The model under review builds one solid part; all positions refer to its coordinate system, in mm. Face numbers are marked on the shaded views. A direction names the side the tool comes from. Round coordinates to 2 decimals unless told otherwise and drop trailing zeros. Order: outer loops, then holes, each group sorted by start corner. A loop starts at its lowest first (then second) coordinate and runs counter-clockwise, first axis right, second up.
```python
from build123d import *

# Parameters (mm, degrees)
F1_DEPTH = 12
F3_DEPTH = 10
F4_W     = 12
F4_H     = 7.5
F5_DEPTH = 10


with BuildPart() as f1:
    # F0 (on Top) → F1 (new body)
    with BuildSketch(Plane.XY):
        with BuildLine():
            Line((-12.672, -19.5), (11.5, -19.5))
            ThreePointArc((11.5, -19.5), (17.156854, -17.156854), (19.5, -11.5))
            Line((19.5, -11.5), (19.5, 11.5))
            ThreePointArc((19.5, 11.5), (17.156854, 17.156854), (11.5, 19.5))
            Line((11.5, 19.5), (-12.672, 19.5))
            ThreePointArc((-12.672, 19.5), (-17.500125, 17.500125), (-19.5, 12.672))
            Line((-19.5, 12.672), (-19.5, -12.672))
            ThreePointArc((-19.5, -12.672), (-17.500125, -17.500125), (-12.672, -19.5))
        make_face()
    extrude(amount=F1_DEPTH)

    # F2 (on face) → F3 (cut)
    with BuildSketch(Plane.XY.offset(12)):
        with BuildLine():
            Line((-10.672, -17.5), (9.5, -17.5))
            ThreePointArc((9.5, -17.5), (15.156854, -15.156854), (17.5, -9.5))
            Line((17.5, -9.5), (17.5, 9.5))
            ThreePointArc((17.5, 9.5), (15.156854, 15.156854), (9.5, 17.5))
            Line((9.5, 17.5), (-10.672, 17.5))
            ThreePointArc((-10.672, 17.5), (-15.500125, 15.500125), (-17.5, 10.672))
            Line((-17.5, 10.672), (-17.5, -10.672))
            ThreePointArc((-17.5, -10.672), (-15.500125, -15.500125), (-10.672, -17.5))
        make_face()
    extrude(amount=-F3_DEPTH, mode=Mode.SUBTRACT)

    # F4 (on face) → F5 (cut)
    with BuildSketch(Plane.YZ.offset(19.5)):
        with Locations((-5.2, 5.004)):
            Rectangle(F4_W, F4_H)
    extrude(amount=-F5_DEPTH, mode=Mode.SUBTRACT)


solid = f1.part
```
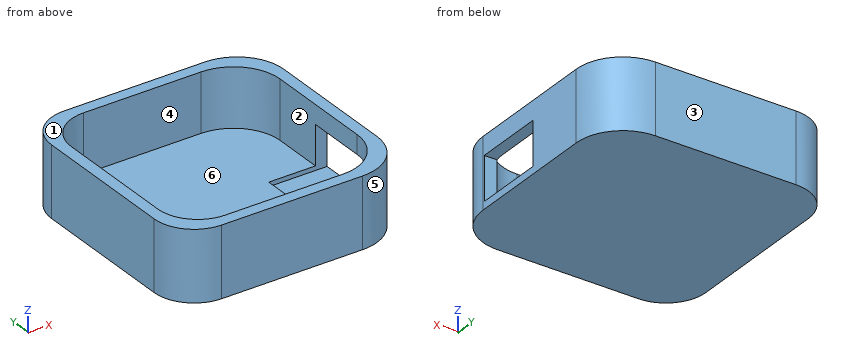
(1) Draft analysis for pull direction Y (two halves, no side actions). For the marked faces 1, 2, 3 and 4, state which applies: pulls with the +Y half, pulls with the -Y half, needs draft (parallel to the pull), parting line crosses it, or undercut.
Data:
face 1: needs draft
face 2: undercut
face 3: pulls with the +Y half
face 4: undercut
(2) To check wall thickness, follow probe 1 along Y at (x, z) = (3, 6); probe 2 along Z at (x, y) = (15.5, 12.5). State the ranges of each line that lie inside material, in increasing order.
Data:
probe 1: y = -19.5 to -17.5, 17.5 to 19.5
probe 2: z = 0 to 2
(3) Consider section C-C (z = 4). Write out the cut boundary in (x, y), and give its area (3 significant figures).
Data:
outline: (-19.5, -12.67) arc R6.83 ccw to (-12.67, -19.5) - (11.5, -19.5) arc R8 ccw to (19.5, -11.5) - (19.5, -11.2) - (17.32, -11.2) arc R8 cw to (9.5, -17.5) - (-10.67, -17.5) arc R6.83 cw to (-17.5, -10.67) - (-17.5, 10.67) arc R6.83 cw to (-10.67, 17.5) - (9.5, 17.5) arc R8 cw to (17.5, 9.5) - (17.5, 0.8) - (19.5, 0.8) - (19.5, 11.5) arc R8 ccw to (11.5, 19.5) - (-12.67, 19.5) arc R6.83 ccw to (-19.5, 12.67) - close
area: 272 mm2
(4) Consider section A-A (x = -4.5). Write out the cut boundary in (y, z), and give its area (3 significant figures).
Data:
outline: (-19.5, 0) - (19.5, 0) - (19.5, 12) - (17.5, 12) - (17.5, 2) - (-17.5, 2) - (-17.5, 12) - (-19.5, 12) - close
area: 118 mm2
(5) Consider section B-B (y = -2). Write out the cut boundary in (x, z), and give its area (3 significant figures).
Data:
outline: (-19.5, 0) - (19.5, 0) - (19.5, 1.25) - (9.5, 1.25) - (9.5, 2) - (-17.5, 2) - (-17.5, 12) - (-19.5, 12) - close; (17.5, 8.75) - (19.5, 8.75) - (19.5, 12) - (17.5, 12) - close
area: 97.0 mm2
(6) Insertion check: pin 1 (3 mm diameter, centred on x = -6, y = 8.5, fed in from -Z); pin 2 (10.5 mm diameter, centred on x = 1, y = -0.5, fed in from +Z); pin 3 (4 mm diameter, centred on x = 16, z = 6.5, fed in from -Y). Each pin has a flat end and moves straight along its axis. Give the tip position at first contact, or say it passes through.
Data:
pin 1: stops at z = 0
pin 2: stops at z = 2
pin 3: stops at y = -19.1
(7) For the marked faces 5 and 6, list the 3-axis set-ups (+Z, -Z, +X, -X, +Y, -Y) from which the entire face can be reached by the end or side of a thin tool; tool diameter is ignored.
Data:
face 5: +Z, -Z, +X, -Y
face 6: +Z
